```python
from build123d import *

# Parameters (mm, degrees)
SKETCH1_W                      = 100
SKETCH1_H                      = 100
SKETCH1_W_2                    = 94
SKETCH1_H_2                    = 94
EXTRUDE_THIN1_DEPTH            = 130
FILLET1_R                      = 0.5
FILLET2_R                      = 3
F_8_0_8_DIAMETER_HOLE2_D       = 8
F_8_0_8_DIAMETER_HOLE3_D       = 8
F_10_0_10_DIAMETER_HOLE1_D     = 10
F_10_0_10_DIAMETER_HOLE2_D     = 10
M8X1_25_TAPPED_HOLE1_D         = 6.8
M8X1_25_TAPPED_HOLE1_DEPTH     = 3
M8X1_25_TAPPED_HOLE2_D         = 6.8
M8X1_25_TAPPED_HOLE2_DEPTH     = 3
F_10_0_10_DIAMETER_HOLE3_D     = 10
F_10_0_10_DIAMETER_HOLE3_DEPTH = 3
F_6_0_6_DIAMETER_HOLE1_D       = 6
F_6_0_6_DIAMETER_HOLE1_DEPTH   = 3
F_10_0_10_DIAMETER_HOLE4_D     = 10
F_10_0_10_DIAMETER_HOLE4_DEPTH = 3


with BuildPart() as part:
    # Sketch1 → Extrude-Thin1 (new body)
    with BuildSketch(Plane.XY):
        Rectangle(SKETCH1_W, SKETCH1_H)
        Rectangle(SKETCH1_W_2, SKETCH1_H_2, mode=Mode.SUBTRACT)
    extrude(amount=EXTRUDE_THIN1_DEPTH)

    # Fillet1
    fillet1_edges = [part.edges().sort_by_distance(p)[0] for p in [
        (47, -47, 65),
        (47, 47, 65),
        (-47, 47, 65),
        (-47, -47, 65),
    ]]
    fillet(fillet1_edges, radius=FILLET1_R)

    # Fillet2
    fillet2_edges = [part.edges().sort_by_distance(p)[0] for p in [
        (50, -50, 65),
        (-50, -50, 65),
        (-50, 50, 65),
        (50, 50, 65),
    ]]
    fillet(fillet2_edges, radius=FILLET2_R)

    # Ø8.0 (8) Diameter Hole2 (through all)
    with Locations(Plane(origin=(0, 50, 0), x_dir=(1, 0, 0), z_dir=(0, 1, 0))):
        with Locations((28, -32), (28, -90)):
            Hole(F_8_0_8_DIAMETER_HOLE2_D / 2)

    # Ø8.0 (8) Diameter Hole3 (through all)
    with Locations(Plane(origin=(50, 0, 0), x_dir=(0, 0, -1), z_dir=(1, 0, 0))):
        with Locations((-14, 31), (-110, 31)):
            Hole(F_8_0_8_DIAMETER_HOLE3_D / 2)

    # Ø10.0 (10) Diameter Hole1 (through all)
    with Locations(Plane(origin=(0, 50, 0), x_dir=(1, 0, 0), z_dir=(0, 1, 0))):
        with Locations((-34, -56)):
            Hole(F_10_0_10_DIAMETER_HOLE1_D / 2)

    # Ø10.0 (10) Diameter Hole2 (through all)
    with Locations(Plane(origin=(50, 0, 0), x_dir=(0, 0, -1), z_dir=(1, 0, 0))):
        with Locations((-44, -31)):
            Hole(F_10_0_10_DIAMETER_HOLE2_D / 2)

    # M8x1.25 Tapped Hole1
    with Locations(Plane.ZY.offset(50)):
        with Locations((56, -15), (56, 35)):
            Hole(M8X1_25_TAPPED_HOLE1_D / 2, depth=M8X1_25_TAPPED_HOLE1_DEPTH)

    # M8x1.25 Tapped Hole2
    with Locations(Plane(origin=(0, -50, 0), x_dir=(-1, 0, 0), z_dir=(0, -1, 0))):
        with Locations((20, -44), (-35, -44)):
            Hole(M8X1_25_TAPPED_HOLE2_D / 2, depth=M8X1_25_TAPPED_HOLE2_DEPTH)

    # Ø10.0 (10) Diameter Hole3
    with Locations(Plane(origin=(50, 0, 0), x_dir=(0, 0, -1), z_dir=(1, 0, 0))):
        with Locations((-70, 0)):
            Hole(F_10_0_10_DIAMETER_HOLE3_D / 2, depth=F_10_0_10_DIAMETER_HOLE3_DEPTH)

    # Ø6.0 (6) Diameter Hole1
    with Locations(Plane(origin=(50, 0, 0), x_dir=(0, 0, -1), z_dir=(1, 0, 0))):
        with Locations((-41.157258279, -16.652364697), (-53.347635303, 28.842741721), (-98.842741721, 16.652364697), (-86.652364697, -28.842741721)):
            Hole(F_6_0_6_DIAMETER_HOLE1_D / 2, depth=F_6_0_6_DIAMETER_HOLE1_DEPTH)

    # Ø10.0 (10) Diameter Hole4
    with Locations(Plane(origin=(0, 50, 0), x_dir=(1, 0, 0), z_dir=(0, 1, 0))):
        with Locations((-3, -105)):
            Hole(F_10_0_10_DIAMETER_HOLE4_D / 2, depth=F_10_0_10_DIAMETER_HOLE4_DEPTH)


solid = part.part
```
Model file for the job. Use its own axes, mm. A direction names the side the tool comes from. Coordinates: 2 decimals unless noted, no trailing zeros. Write each loop counter-clockwise with the first axis right and the second up, starting at its lowest first coordinate (ties: lowest second). Pieces come first, ordered by that corner, then holes. Notation, with made-up numbers: (17, 47.5) - (28, 47.5) arc R23 cw to (28, 85.5) - close; hole circle Ø5 at (37.25, 20.5). An arc over 180 degrees is marked (long way). Use a Markdown table: item, result. Add a question column.
Item 1: Band-saw the part on D-D, the plane x = 16.5. Write the cut outline in (y, z).
Item 2: Drill centre lines: line 1 along X through (y, z) = (-40, 40); line 2 along Z through (x, y) = (-3, 49.35). Where is each one in solid material? Low to high.
Item 3: Drop a flat-ended pin along its axis: pin 1 (6 mm diameter, centred on x = -20, z = 44, fed in from -Y). Give the stop position or say it passes through.
Item 4: Band-saw the part on C-C, the plane z = 32. Write the cut outline in (x, y), and give its area (3 significant figures).
Item 5: 3-axis set-ups, long thin cutter, end or side, ignore diameter. For faces 4 (the face through (47, -1, 64)), 5 (the face through (-18.172, -48.479, 41.133)), 6 (the face through (48.479, 17.553, 101.704)), 7 (the face through (-48.48, -16.3, 52.86)): which of +Z, -Z, +X, -X, +Y, -Y reach the whole face in a straight line?
Item 6: Band-saw the part on B-B, the plane y = 0. Write the cut outline in (x, z).
Item 7: Two-plate mould, pull along Y, no slides. Class faces 1 (the face through (-1, -50, 64)), 2 (the face through (48.479, -30.668, 84.272)), 3 (the face through (38.14, -48.48, 45.3)): pulls with the +Y half, pulls with the -Y half, needs draft (parallel to the pull), parting line crosses it, or undercut.
Item 8: Band-saw the part on A-A, the plane x = -20. Write the cut outline in (y, z).
A:
| question | item | result |
|---|---|---|
| 1 | outline | (-50, 0) - (-47, 0) - (-47, 130) - (-50, 130) - close; (47, 0) - (50, 0) - (50, 130) - (47, 130) - close |
| 2 | line 1 | x = -50 to -47, 47 to 50 |
| 2 | line 2 | z = 0 to 100, 110 to 130 |
| 3 | pin 1 | stops at y = 47 |
| 4 | outline | (-50, -47) arc R3 ccw to (-47, -50) - (24, -50) - (24, -47) - (-46.5, -47) arc R0.5 cw to (-47, -46.5) - (-47, 46.5) arc R0.5 cw to (-46.5, 47) - (24, 47) - (24, 50) - (-47, 50) arc R3 ccw to (-50, 47) - close; (32, -50) - (47, -50) arc R3 ccw to (50, -47) - (50, 47) arc R3 ccw to (47, 50) - (32, 50) - (32, 47) - (46.5, 47) arc R0.5 cw to (47, 46.5) - (47, -46.5) arc R0.5 cw to (46.5, -47) - (32, -47) - close |
| 4 | area | 1,110 mm² |
| 5 | face 4 | +Z, -Z |
| 5 | face 5 | -Y |
| 5 | face 6 | +X |
| 5 | face 7 | -X |
| 6 | outline | (-50, 0) - (-47, 0) - (-47, 130) - (-50, 130) - close; (47, 0) - (50, 0) - (50, 65) - (47, 65) - close; (47, 75) - (50, 75) - (50, 130) - (47, 130) - close |
| 7 | face 1 | pulls with the -Y half |
| 7 | face 2 | undercut |
| 7 | face 3 | needs draft |
| 8 | outline | (-50, 0) - (-47, 0) - (-47, 40.6) - (-50, 40.6) - close; (-50, 47.4) - (-47, 47.4) - (-47, 130) - (-50, 130) - close; (47, 0) - (50, 0) - (50, 130) - (47, 130) - close |
